Verification items for this drawing (mm, ordinates from the low corner). A direction names the side the tool comes from. Round coordinates to 2 decimals unless told otherwise and drop trailing zeros. Write each loop counter-clockwise with the first axis right and the second up, starting at its lowest first coordinate (ties: lowest second). Pieces come first, ordered by that corner, then holes.
Item 1: Scan lines: probe 1 along Z at (x, y) = (11.1, 7); probe 2 along Z at (x, y) = (17, 15.5) (1 decimal); probe 3 along X at (y, z) = (19, 14.75) (1 decimal). Record each from-to range of solid material in increasing order.
Item 2: Cross-section at D-D (z = 3.25). Enter the section's corners in (x, y) (1 decimal).
Item 3: Depth check by flat-ended pin: P1, Ø3, axis at x = 17, y = 16.5, coming from the -Z side; P2, Ø5.5, axis at x = 4.5, z = 6.5, coming from the +Y side (1 decimal); P3, Ø1.5, axis at x = 9, y = 16.5, coming from the +Z side. Enter the tip coordinate at first touch or a pass-through.
Item 4: Draft check along Z on the marked faces 3, 4 and 5. Enter one of: pulls with the +Z half, pulls with the -Z half, needs draft (parallel to the pull), parting line crosses it, or undercut.
Item 5: Cross-section at B-B (z = 8.5). Enter the section's corners in (x, y) (1 decimal).
Item 6: Cross-section at C-C (y = 2.5). Enter the section's corners in (x, z) (1 decimal).
Item 7: Access from +Z, -Z, +X, -X, +Y, -Y to the whole of each face (thin tool, end or side, straight path). Record for the marked faces 1 and 2.
Item 8: Cross-section at A-A (x = 11.5). Enter the section's corners in (y, z), then the cut area to 3 significant figures.
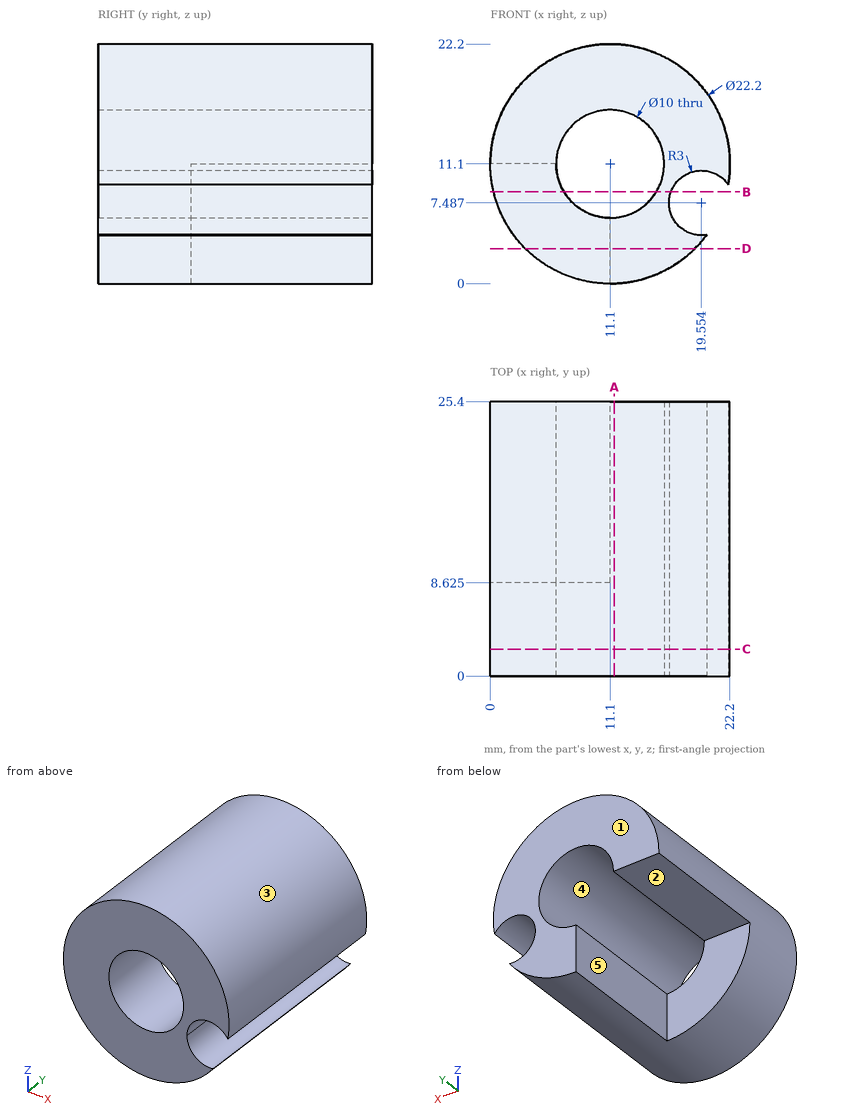
Resolved:
1. probe 1: z = 0 to 6.1, 16.1 to 22.2
1. probe 2: z = 1.7 to 5.9, 9.1 to 20.5
1. probe 3: x = 0.6 to 7.7, 14.5 to 21.6
2. outline: (3.3, 0) - (18.9, 0) - (18.9, 25.4) - (11.1, 25.4) - (11.1, 8.6) - (3.3, 8.6) - close
3. P1: stops at z = 0.91
3. P2: stops at y = 8.6
3. P3: stops at z = 22.12
4. face 3: parting line crosses it
4. face 4: undercut
4. face 5: needs draft
5. outline: (0.3, 0) - (6.8, 0) - (6.8, 8.6) - (0.3, 8.6) - close; (15.4, 0) - (16.7, 0) - (16.7, 25.4) - (15.4, 25.4) - close
6. outline: (20, 4.5) arc R3 cw (long way) to (22, 9.2) arc R11.1 ccw (long way) to start; hole circle Ø10 at (11.1, 11.1)
7. face 1: +Z, -Z, +X, -X, +Y
7. face 2: -Z, -X, +Y
8. outline: (0, 0.01) - (25.4, 0.01) - (25.4, 6.12) - (0, 6.12) - close; (0, 16.08) - (25.4, 16.08) - (25.4, 22.19) - (0, 22.19) - close
8. area: 310 mm2
